The listing builds one solid part. Answer for the finished solid, in the listing's coordinates (mm). A direction names the side the tool comes from. Give positions to 0.01 mm unless a question says otherwise; leave off trailing zeros. Order: outer loops, then holes, each group sorted by start corner. A loop starts at its lowest first (then second) coordinate and runs counter-clockwise, first axis right, second up. Notation, with made-up numbers: (-32, 37.5) - (5, 37.5) arc R27 cw to (5, 72.5) - close; hole circle Ø3 at (51, 32.5). An arc over 180 degrees is marked (long way). Answer in a Markdown table with one row per item.
from build123d import *

# Parameters (mm, degrees)
CROQUIS1_R                   = 10
SALIENTE_EXTRUIR2_DEPTH      = 102
CROQUIS2_R                   = 5.5
SALIENTE_EXTRUIR3_DEPTH      = 1.5
SALIENTE_EXTRUIR3_DEPTH_BACK = 103.5


with BuildPart() as part:
    # Croquis1 → Saliente-Extruir2 (new body)
    with BuildSketch(Plane.XY):
        Circle(CROQUIS1_R)
    extrude(amount=SALIENTE_EXTRUIR2_DEPTH)

    # Croquis2 → Saliente-Extruir3 (add, two sides)
    with BuildSketch(Plane.XY.offset(102)) as saliente_extruir3_sk:
        Circle(CROQUIS2_R)
    extrude(amount=SALIENTE_EXTRUIR3_DEPTH)
    extrude(saliente_extruir3_sk.sketch, amount=-SALIENTE_EXTRUIR3_DEPTH_BACK)


solid = part.part
Item 1: Which of the six approach directions +Z, -Z, +X, -X, +Y, -Y give full straight-line access (tool end or side, diameter ignored) to faces 1 (the face through (-1.19, -5.37, 102.74)), 2 (the face through (0, 0, 103.5)), 3 (the face through (4, -4, 0))?
Answer block:
| item | result |
|---|---|
| face 1 | +Z |
| face 2 | +Z, +X, -X, +Y, -Y |
| face 3 | -Z |
Item 2: Consider line 1 (Z direction, x = 5, y = -5.25); line 2 (X direction, y = 3.75, z = 12); line 3 (X direction, y = -8.25, z = 20.5). Determine where each line is inside the solid, lowest interval first.
Answer block:
| item | result |
|---|---|
| line 1 | 0 to 102 |
| line 2 | -9.27 to 9.27 |
| line 3 | -5.65 to 5.65 |
Item 3: Each of these flat-tipped pins is pushed along its axis until it touches: P1, Ø4, axis at y = 4.5, z = 30.5, coming from the +X side; P2, Ø4, axis at x = 7.5, z = 85.5, coming from the +Y side; P3, Ø1.5, axis at x = 6, z = 79, coming from the -Y side. Where does it stop, or does it pass through?
Answer block:
| item | result |
|---|---|
| P1 | x = 9.68 |
| P2 | y = 8.35 |
| P3 | y = -8.51 |
Item 4: Find section A-A on x = -3.5. Write down the section's boundary in (y, z).
Answer block:
| item | result |
|---|---|
| outline | (-9.37, 0) - (-4.24, 0) - (-4.24, -1.5) - (4.24, -1.5) - (4.24, 0) - (9.37, 0) - (9.37, 102) - (4.24, 102) - (4.24, 103.5) - (-4.24, 103.5) - (-4.24, 102) - (-9.37, 102) - close |
Item 5: Find section D-D on x = 8. Write down the section's boundary in (y, z).
Answer block:
| item | result |
|---|---|
| outline | (-6, 0) - (6, 0) - (6, 102) - (-6, 102) - close |
Item 6: Find section B-B on z = 77.5. Write down the section's boundary in (x, y).
Answer block:
| item | result |
|---|---|
| outline | circle Ø20 at (0, 0) |
